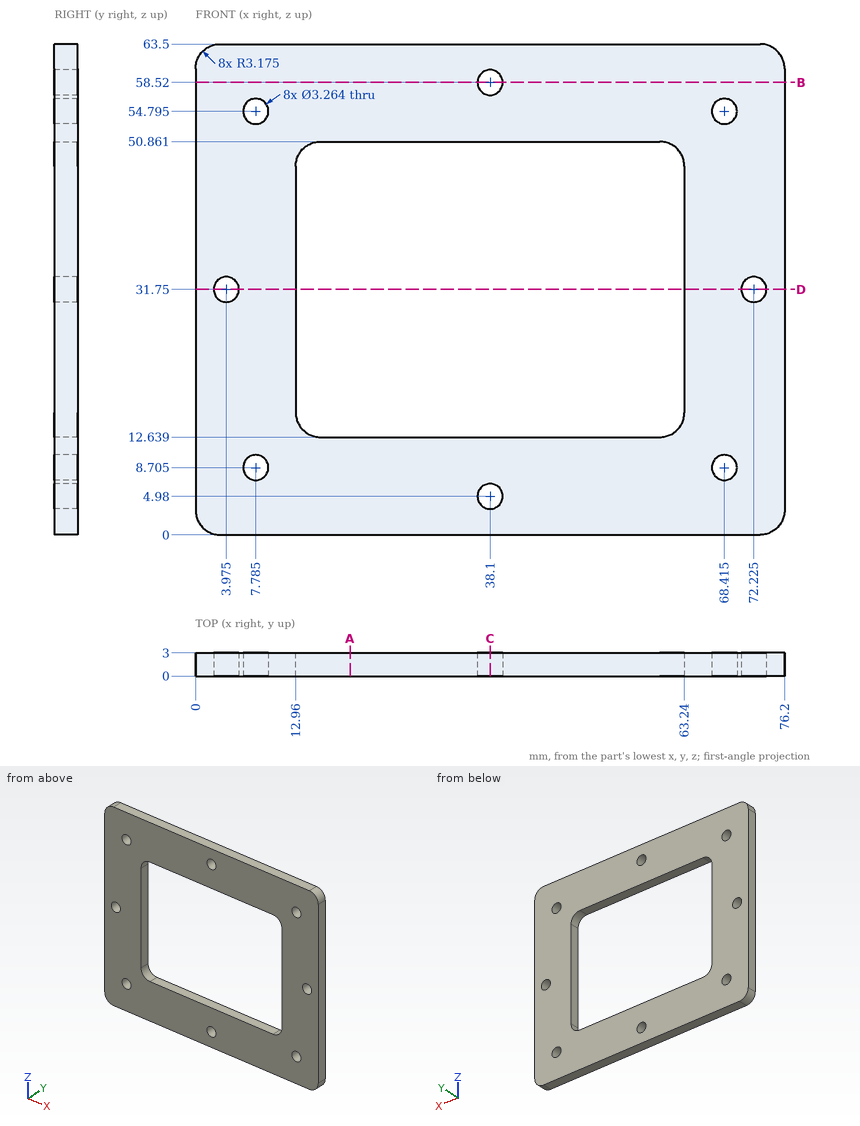
Geometry check sheet. Reference: drawing and pictorial views, mm from the part's lowest x, y, z. Give positions to 0.01 mm unless a question says otherwise; leave off trailing zeros. Loops run counter-clockwise (first coordinate to the right, second up) from the corner with the lowest first, then second, coordinate; pieces in that order, holes last. Notation, with made-up numbers: (-15, 25) -> (13, 25) arc R14 ccw to (13, 33) -> close; hole circle Ø10 at (88, 34.5). An arc over 180 degrees is marked (long way). Answer in a Markdown table with one row per item. Add a question column.
1) Gauge pin test, flat ends, axial feed: P1, Ø4, axis at x = 7.785, z = 54.795, coming from the -Y side; P2, Ø2, axis at x = 38.1, z = 58.52, coming from the +Y side. Record the tip position at first contact, or that the pin passes through.
2) Cross-section at A-A on x = 20. Record the boundary of the cut face in (y, z).
3) Cross-section at B-B on z = 58.52. Record the boundary of the cut face in (x, y), and give its area (3 significant figures).
4) Cross-section at C-C on x = 38.1. Record the boundary of the cut face in (y, z).
5) Cross-section at D-D on z = 31.75. Record the boundary of the cut face in (x, y).
6) Material ranges on probe 1 along Z at (x, y) = (8, 0.6); probe 2 along Z at (x, y) = (38.1, 1.65); probe 3 along Z at (x, y) = (18, 2.75), recorded low to high. Write a range as from..to.
Outcome:
| question | item | result |
|---|---|---|
| 1 | P1 | stops at y = 0 |
| 1 | P2 | passes through |
| 2 | outline | (0, 0) -> (3, 0) -> (3, 12.64) -> (0, 12.64) -> close; (0, 50.86) -> (3, 50.86) -> (3, 63.5) -> (0, 63.5) -> close |
| 3 | outline | (0, 0) -> (36.47, 0) -> (36.47, 3) -> (0, 3) -> close; (39.73, 0) -> (76.2, 0) -> (76.2, 3) -> (39.73, 3) -> close |
| 3 | area | 219 mm^2 |
| 4 | outline | (0, 0) -> (3, 0) -> (3, 3.35) -> (0, 3.35) -> close; (0, 6.61) -> (3, 6.61) -> (3, 12.64) -> (0, 12.64) -> close; (0, 50.86) -> (3, 50.86) -> (3, 56.89) -> (0, 56.89) -> close; (0, 60.15) -> (3, 60.15) -> (3, 63.5) -> (0, 63.5) -> close |
| 5 | outline | (0, 0) -> (2.34, 0) -> (2.34, 3) -> (0, 3) -> close; (5.61, 0) -> (12.96, 0) -> (12.96, 3) -> (5.61, 3) -> close; (63.24, 0) -> (70.59, 0) -> (70.59, 3) -> (63.24, 3) -> close; (73.86, 0) -> (76.2, 0) -> (76.2, 3) -> (73.86, 3) -> close |
| 6 | probe 1 | z = 0..7.09, 10.32..53.18, 56.41..63.5 |
| 6 | probe 2 | z = 0..3.35, 6.61..12.64, 50.86..56.89, 60.15..63.5 |
| 6 | probe 3 | z = 0..12.64, 50.86..63.5 |
